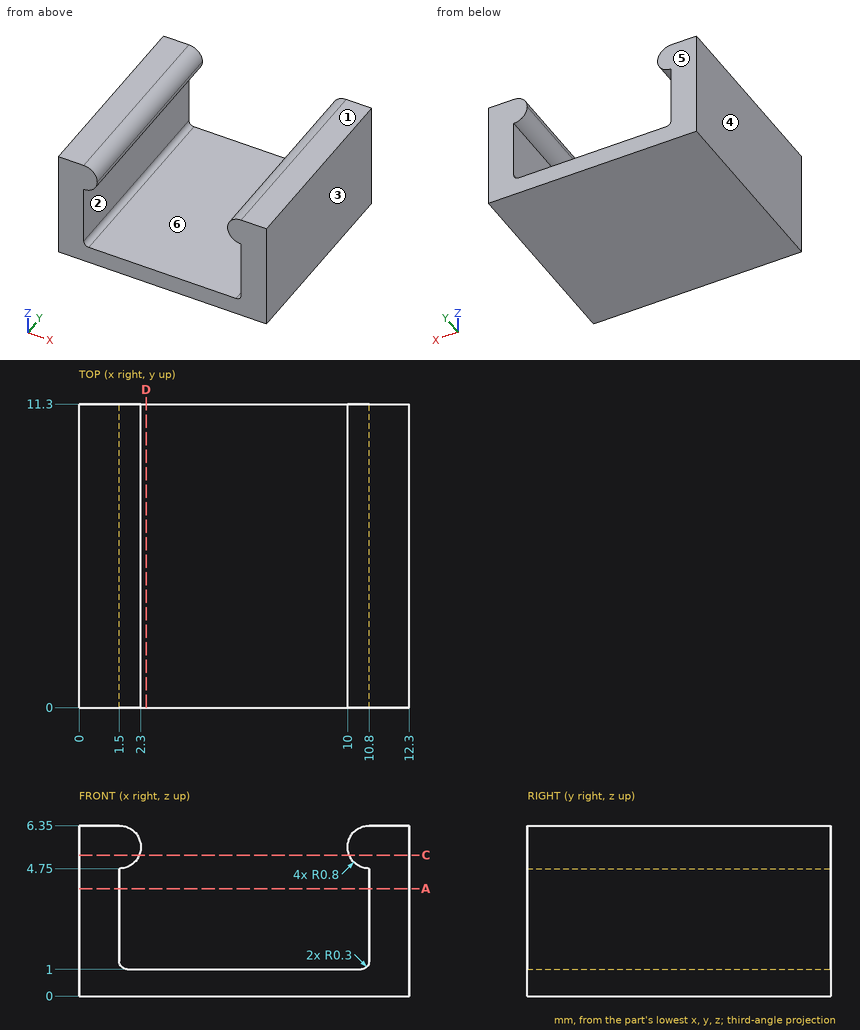
Answer from the drawing. Dimensions are ordinates in mm from the lowest x, y and z of the part. A direction names the side the tool comes from. Give positions to 0.01 mm unless a question says otherwise; leave off trailing zeros. Loops run counter-clockwise (first coordinate to the right, second up) from the corner with the lowest first, then second, coordinate; pieces in that order, holes last. Notation, with made-up numbers: (58.25, -23.75) -> (115.25, -23.75) arc R15 ccw to (115.25, -16.75) -> close; hole circle Ø8 at (48.25, 47). An arc over 180 degrees is marked (long way). Use a Markdown table: item, result.
Q1. Section D-D, the plane x = 2.5 is taken. Determine the outline of the cut face in (y, z).
Solved:
| item | result |
|---|---|
| outline | (0, 0) -> (11.3, 0) -> (11.3, 1) -> (0, 1) -> close |
Q2. A tool of negligible diameter and unlimited length cuts with its end or side. For the marked faces 1 and 2, from which of +Z, -Z, +X, -X, +Y, -Y can it reach the whole face along a straight path? Write none if from no direction.
Solved:
| item | result |
|---|---|
| face 1 | +Z, +X, -X, +Y, -Y |
| face 2 | +Y, -Y |
Q3. Section C-C, the plane z = 5.25 is taken. Determine the outline of the cut face in (x, y), then the cut area to 3 significant figures.
Solved:
| item | result |
|---|---|
| outline | (0, 0) -> (2.24, 0) -> (2.24, 11.3) -> (0, 11.3) -> close; (10.06, 0) -> (12.3, 0) -> (12.3, 11.3) -> (10.06, 11.3) -> close |
| area | 50.7 mm^2 |
Q4. Determine the mould class of the marked faces 3, 4, 5 and 6 for opening direction X: pulls with the +X half, pulls with the -X half, needs draft (parallel to the pull), parting line crosses it, or undercut.
Solved:
| item | result |
|---|---|
| face 3 | pulls with the +X half |
| face 4 | pulls with the -X half |
| face 5 | needs draft |
| face 6 | undercut |
Q5. Find the intervals of material crossed by line 1 along X through (y, z) = (1.5, 3); line 2 along X through (y, z) = (5, 5.5); line 3 along Z through (x, y) = (7.5, 9), in increasing order.
Solved:
| item | result |
|---|---|
| line 1 | x = 0 to 1.5, 10.8 to 12.3 |
| line 2 | x = 0 to 2.3, 10 to 12.3 |
| line 3 | z = 0 to 1 |
Q6. Section A-A, the plane z = 4 is taken. Determine the outline of the cut face in (x, y), then the cut area to 3 significant figures.
Solved:
| item | result |
|---|---|
| outline | (0, 0) -> (1.5, 0) -> (1.5, 11.3) -> (0, 11.3) -> close; (10.8, 0) -> (12.3, 0) -> (12.3, 11.3) -> (10.8, 11.3) -> close |
| area | 33.9 mm^2 |
